CAD build for the part. Positions are in the model's coordinates, mm. A direction names the side the tool comes from. Round coordinates to 2 decimals unless told otherwise and drop trailing zeros. Loops run counter-clockwise (first coordinate to the right, second up) from the corner with the lowest first, then second, coordinate; pieces in that order, holes last. Notation, with made-up numbers: (-31, 0) - (-11, 0) arc R24 cw to (-11, 19) - close; hole circle Ø6 at (24.5, -39). An arc over 180 degrees is marked (long way). One line per question, with ' | ' between items.
```python
from build123d import *

# Parameters (mm, degrees)
SKETCH1_W           = 7.1
SKETCH1_H           = 7
BOSS_EXTRUDE1_DEPTH = 6.55
SKETCH2_W           = 0.3
SKETCH2_H           = 0.3
SKETCH2_W_2         = 1
SKETCH2_H_2         = 0.4
BOSS_EXTRUDE2_DEPTH = 3.5
SKETCH3_W           = 2.95
SKETCH3_H           = 5.612486488
CUT_EXTRUDE1_DEPTH  = 13.874587372
SKETCH4_R           = 1.55
BOSS_EXTRUDE3_DEPTH = 5.85


with BuildPart() as part:
    # Sketch1 → Boss-Extrude1 (new body)
    with BuildSketch(Plane(origin=(0, 0, 0), x_dir=(0, 0, -1), z_dir=(1, 0, 0))):
        Rectangle(SKETCH1_W, SKETCH1_H)
    extrude(amount=-BOSS_EXTRUDE1_DEPTH)

    # Sketch2 → Boss-Extrude2 (add)
    with BuildSketch(Plane.XZ.offset(3.5)):
        with Locations((-2.55, 2.25)):
            Rectangle(SKETCH2_W, SKETCH2_H)
        with Locations((-5.05, 3.35)):
            Rectangle(SKETCH2_W_2, SKETCH2_H_2)
    boss_extrude2 = extrude(amount=BOSS_EXTRUDE2_DEPTH)

    # Mirror1: Boss-Extrude2 across plane
    add(boss_extrude2.mirror(Plane.XY))

    # Sketch3 → Cut-Extrude1 (cut, through all)
    with BuildSketch(Plane(origin=(0, 3.5, 0), x_dir=(1, 0, 0), z_dir=(0, 1, 0))):
        with Locations((-5.075, 0.013867293)):
            Rectangle(SKETCH3_W, SKETCH3_H)
    extrude(amount=-CUT_EXTRUDE1_DEPTH, mode=Mode.SUBTRACT)

    # Sketch4 → Boss-Extrude3 (add)
    with BuildSketch(Plane(origin=(0, 0, 0), x_dir=(0, 0, -1), z_dir=(1, 0, 0))):
        with Locations(Location((0, 0.5, 0), (0, 0, 180))):
            Circle(SKETCH4_R)
    extrude(amount=BOSS_EXTRUDE3_DEPTH)


solid = part.part
```
(1) Cut at D-D, the plane x = 5.25. Write the cut outline in (y, z).
Results found:
outline: circle Ø3.1 at (0.5, 0)
(2) Probe L1, parallel to Z at x = -5.5, y = -1; L2, parallel to X at y = -3, z = 2; L3, parallel to Y at x = -3.5, z = -3. List the from-to ranges inside material, lowest first.
Results found:
L1: z = -3.55 to -2.82, 2.79 to 3.55 | L2: x = -3.6 to 0 | L3: y = -3.5 to 3.5
(3) Cut at A-A, the plane y = -5.5. Write the cut outline in (x, z).
Results found:
outline: (-5.55, -3.55) - (-4.55, -3.55) - (-4.55, -3.15) - (-5.55, -3.15) - close; (-5.55, 3.15) - (-4.55, 3.15) - (-4.55, 3.55) - (-5.55, 3.55) - close; (-2.7, -2.4) - (-2.4, -2.4) - (-2.4, -2.1) - (-2.7, -2.1) - close; (-2.7, 2.1) - (-2.4, 2.1) - (-2.4, 2.4) - (-2.7, 2.4) - close
(4) Drop a flat-ended pin along its axis: P1, Ø4, axis at x = 2.5, z = 2.5, coming from the -Y side. Give the stop position or say it passes through.
Results found:
P1: stops at y = -0.97
(5) Two-plate mould, pull along Z, no slides. Class faces 4 (the face through (-3, 3.5, 0)), 5 (the face through (2.884, 1.875, 0.715)), 6 (the face through (-3.6, 0, 0)), 7 (the face through (-5, 0, -2.82)): released by +Z, released by -Z, zero draft, split by the parting line, or undercut.
Results found:
face 4: zero draft | face 5: split by the parting line | face 6: undercut | face 7: undercut
(6) Cut at B-B, the plane z = 0. Write the cut outline in (x, y).
Results found:
outline: (-3.6, -3.5) - (0, -3.5) - (0, -1.05) - (5.85, -1.05) - (5.85, 2.05) - (0, 2.05) - (0, 3.5) - (-3.6, 3.5) - close
(7) Tool access for faces 1 (the face through (0, -2, 0)), 2 (the face through (-5, -5, 3.15)), 3 (the face through (-5, 0, 2.792)): list every direction of +Z, -Z, +X, -X, +Y, -Y with a clear straight run to the whole face (end or side of a thin tool).
Results found:
face 1: +X | face 2: +X, -X, -Y | face 3: -X, +Y, -Y
(8) Cut at C-C, the plane y = -2.75. Write the cut outline in (x, z).
Results found:
outline: (-6.55, -3.55) - (0, -3.55) - (0, 3.55) - (-6.55, 3.55) - (-6.55, 2.79) - (-3.6, 2.79) - (-3.6, -2.82) - (-6.55, -2.82) - close
